Here's how the part is built. I have some questions about the finished solid (model axes, mm). Face numbers are marked on the shaded views. A direction names the side the tool comes from. Coordinates: 2 decimals unless noted, no trailing zeros. Loops run counter-clockwise (first coordinate to the right, second up) from the corner with the lowest first, then second, coordinate; pieces in that order, holes last. Notation, with made-up numbers: (63.25, -22.75) -> (107.25, -22.75) arc R31 cw to (107.25, 10.25) -> close; hole circle Ø5 at (-16.5, 56). An arc over 180 degrees is marked (long way). Answer as a JSON object with one key per item and string values. Group by question number.
Q1. Thinking about a two-plate mould opening in Y: for the marked faces 5, 6, 7 and 8, which applies, released by +Y, released by -Y, zero draft, split by the parting line, or undercut?
Q2. I'm going to push flat-ended pins straight in: pin 1 (0.7 mm diameter, centred on y = 28, z = 2, fed in from -X); pin 2 (1.5 mm diameter, centred on y = 31, z = 1.5, fed in from +X); pin 3 (1.5 mm diameter, centred on x = -48.5, z = 1.5, fed in from +Y); pin 4 (5 mm diameter, centred on x = -54.5, y = 37.5, fed in from -Z). Where does each tip first touch, or does it pass through?
Q3. I want a section at A-A on y = 27.5. Write out the boundary of the cut face in (x, z), then the cut area to 3 significant figures.
Q4. I want a section at D-D on x = -53.75. Write out the boundary of the cut face in (y, z).
Q5. On a 3-axis mill with a long thin cutter (end or side, diameter ignored), from which of +Z, -Z, +X, -X, +Y, -Y can I reach the whole of each face in a straight line? I mean the marked faces 1, 2, 3 and 4. Say none if no direction works.
Q6. I want a section at C-C on z = 2.05. Write out the boundary of the cut face in (x, y), then the cut area to 3 significant figures.
Q7. I want a section at B-B on x = -55.25. Write out the boundary of the cut face in (y, z), then the cut area to 3 significant figures.
Q8. I need wall thicknesses on line 1 (Y direction, x = -53.5, z = 1.1); line 2 (X direction, y = 29, z = 0.15); line 3 (X direction, y = 33.5, z = 2.1). Which ranges of each line are inside material? Lowest first, please.
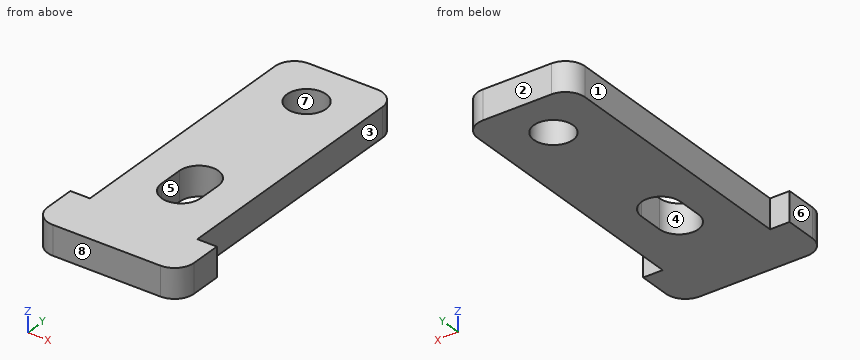
```python
from build123d import *

# Parameters (mm, degrees)
SKETCH_R    = 2
PAD_DEPTH   = 3
FILLET_R    = 2
FILLET001_R = 2
FILLET002_R = 2
FILLET003_R = 2


with BuildPart() as part:
    # Sketch → Pad (new body)
    with BuildSketch(Plane.XY):
        Polygon((-48.942066, 48.928535), (-59.942066, 48.928535), (-59.942066, 20.928535), (-61.942066, 20.928535), (-61.942066, 15.728535), (-46.942066, 15.728535), (-46.942066, 20.928535), (-48.942066, 20.928535), align=None)
        with Locations((-54.519871, 43.928535)):
            Circle(SKETCH_R, mode=Mode.SUBTRACT)
        with BuildLine():
            ThreePointArc((-52.549564, 28.83341), (-54.549564, 30.83341), (-56.549564, 28.83341))
            Line((-56.549564, 28.83341), (-56.549564, 26.340669))
            ThreePointArc((-56.549564, 26.340669), (-54.549564, 24.340669), (-52.549564, 26.340669))
            Line((-52.549564, 28.83341), (-52.549564, 26.340669))
        make_face(mode=Mode.SUBTRACT)
    extrude(amount=PAD_DEPTH)

    # Fillet
    fillet_edges = [part.edges().sort_by_distance(p)[0] for p in [
        (-48.942066, 48.928535, 1.5),
    ]]
    fillet(fillet_edges, radius=FILLET_R)

    # Fillet001
    fillet001_edges = [part.edges().sort_by_distance(p)[0] for p in [
        (-46.942066, 15.728535, 1.5),
    ]]
    fillet(fillet001_edges, radius=FILLET001_R)

    # Fillet002
    fillet002_edges = [part.edges().sort_by_distance(p)[0] for p in [
        (-61.942066, 15.728535, 1.5),
    ]]
    fillet(fillet002_edges, radius=FILLET002_R)

    # Fillet003
    fillet003_edges = [part.edges().sort_by_distance(p)[0] for p in [
        (-59.942066, 48.928535, 1.5),
    ]]
    fillet(fillet003_edges, radius=FILLET003_R)


solid = part.part
```
Result set:
{
 "1": {"face 5": "undercut", "face 6": "zero draft", "face 7": "undercut", "face 8": "released by -Y"},
 "2": {"pin 1": "stops at x = -59.94", "pin 2": "stops at x = -48.94", "pin 3": "stops at y = 47.99", "pin 4": "stops at z = 0"},
 "3": {"outline": "(-59.94, 0) -> (-56.55, 0) -> (-56.55, 3) -> (-59.94, 3) -> close; (-52.55, 0) -> (-48.94, 0) -> (-48.94, 3) -> (-52.55, 3) -> close", "area": "21.0 mm²"},
 "4": {"outline": "(15.73, 0) -> (24.51, 0) -> (24.51, 3) -> (15.73, 3) -> close; (30.67, 0) -> (42.08, 0) -> (42.08, 3) -> (30.67, 3) -> close; (45.77, 0) -> (48.93, 0) -> (48.93, 3) -> (45.77, 3) -> close"},
 "5": {"face 1": "+Z, -Z, -X, +Y", "face 2": "+Z, -Z, +X, -X, +Y", "face 3": "+Z, -Z, +X, +Y", "face 4": "+Z, -Z"},
 "6": {"outline": "(-61.94, 17.73) arc R2 ccw to (-59.94, 15.73) -> (-48.94, 15.73) arc R2 ccw to (-46.94, 17.73) -> (-46.94, 20.93) -> (-48.94, 20.93) -> (-48.94, 46.93) arc R2 ccw to (-50.94, 48.93) -> (-57.94, 48.93) arc R2 ccw to (-59.94, 46.93) -> (-59.94, 20.93) -> (-61.94, 20.93) -> close; hole (-56.55, 26.34) arc R2 ccw to (-52.55, 26.34) -> (-52.55, 28.83) arc R2 ccw to (-56.55, 28.83) -> close; hole circle Ø4 at (-54.52, 43.93)", "area": "347 mm²"},
 "7": {"outline": "(15.73, 0) -> (24.47, 0) -> (24.47, 3) -> (15.73, 3) -> close; (30.71, 0) -> (42.07, 0) -> (42.07, 3) -> (30.71, 3) -> close; (45.79, 0) -> (48.93, 0) -> (48.93, 3) -> (45.79, 3) -> close", "area": "69.7 mm²"},
 "8": {"line 1": "y = 15.73 to 24.64, 30.54 to 42.21, 45.65 to 48.93", "line 2": "x = -59.94 to -56.54, -52.56 to -48.94", "line 3": "x = -59.94 to -48.94"}
}
